Input: part model. Units: mm. Frame: model coordinates. Round coordinates to 2 decimals unless told otherwise and drop trailing zeros. Write each loop counter-clockwise with the first axis right and the second up, starting at its lowest first coordinate (ties: lowest second). Pieces come first, ordered by that corner, then holes. Notation, with made-up numbers: (36.5, 59) - (54.5, 59) arc R25 ccw to (54.5, 95) - close; hole circle Ø2 at (-18.75, 5). An arc over 180 degrees is marked (long way). Use one line per item in the form item = value.
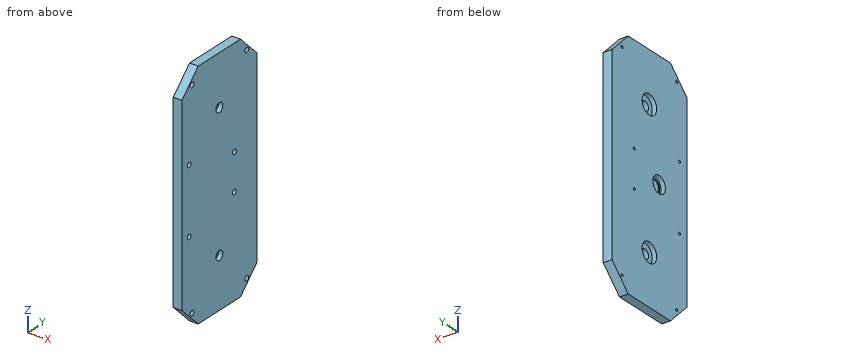
Autodesk Inventor part; units mm, degrees
ref_plane "YZ Plane" through (0, 0, 0) normal (1, 0, 0) x (0, 1, 0)
ref_plane "XZ Plane" through (0, 0, 0) normal (0, 1, 0) x (-1, 0, 0)
ref_plane "XY Plane" through (0, 0, 0) normal (0, 0, 1) x (1, 0, 0)
sketch "Sketch1" plane through (0, 0, 0) normal (1, 0, 0) x (0, 1, 0)
  line L0 (-57.5, 135) -> (57.5, 135)
  line L1 (57.5, 135) -> (57.5, -135)
  line L2 (57.5, -135) -> (-57.5, -135)
  line L3 (-57.5, -135) -> (-57.5, 135)
  line L4 (-57.5, 135) -> (57.5, -135) construction
  line L5 (57.5, 135) -> (-57.5, -135) construction
  circle A0 centre (0, 77.5) radius 5.3
  circle A1 centre (0, -77.5) radius 5.3
  circle A2 centre (0, 0) radius 5.3
  line L6 (0, 77.5) -> (0, -77.5) construction
  line L7 (51.5, -129) -> (51.5, 129)
  line L8 (51.5, 129) -> (-51.5, 129)
  line L9 (-51.5, 129) -> (-51.5, -129)
  line L10 (-51.5, -129) -> (51.5, -129)
  dimension "d0" = 155
  dimension "d1" = 10.6
  dimension "d2" = 270
  dimension "d3" = 115
  dimension "d4" = 6
extrude "Extrusion1" add sketch "Sketch1" along normal blind 10 contours L0 L1 L2 L3 | A2 | L10 L9 L8 L7
chamfer "Chamfer2" distance 25 angle 45 4 edges at (5, 57.5, -135) (5, -57.5, -135) (5, -57.5, 135) (5, 57.5, 135)
sketch "Sketch11" plane through (0, 0, 0) normal (-1, 0, 0) x (0, 0, 1)
  circle A0 centre (-77.5, 0) radius 5.3
  circle A1 centre (77.5, 0) radius 5.3
  circle A2 centre (-77.5, 0) radius 11.15
  circle A3 centre (77.5, 0) radius 11.15
  point P0 (0, 0)
  dimension "d41" = 22.3
extrude "Extrusion10" cut sketch "Sketch11" against normal blind 5 contours A0 | A1 | A2 | A3
sketch "Sketch12" plane through (0, 0, 0) normal (-1, 0, 0) x (0, 0, 1)
  circle A0 centre (0, -15) radius 9.65
  point P0 (0, 0)
  dimension "d44" = 15
  dimension "d45" = 19.3
extrude "Extrusion11" cut sketch "Sketch12" against normal blind 5
sketch "Sketch13" plane through (5, -15, 0) normal (-1, 0, 0) x (0, 0, 1)
  circle A0 centre (0, 0) radius 9.65
  circle A1 centre (0, 0) radius 7.5
  point P0 (0, 15)
  dimension "d48" = 15
extrude "Extrusion12" cut sketch "Sketch13" against normal blind 1 contours A1
sketch "Sketch14" plane through (10, 0, 0) normal (1, 0, 0) x (0, 0, -1)
  circle A0 centre (-119.5, 42) radius 1.5
  circle A1 centre (-119.5, -42) radius 1.5
  circle A2 centre (-37.6476, -46.4615) radius 1.5
  circle A3 centre (37.6476, -46.4615) radius 1.5
  circle A4 centre (-21.0923, 23.1558) radius 1.5
  circle A5 centre (21.0923, 23.1558) radius 1.5
  circle A6 centre (119.5, -42) radius 1.5
  circle A7 centre (119.5, 42) radius 1.5
  point P0 (0, 0)
extrude "Extrusion13" cut sketch "Sketch14" against normal through all
sketch "Sketch15" plane through (10, 0, 0) normal (1, 0, 0) x (0, 0, -1)
  circle A0 centre (-21.0923, 23.1558) radius 1.5
  circle A1 centre (119.5, -42) radius 1.5
  circle A2 centre (-119.5, -42) radius 1.5
  circle A3 centre (37.6476, -46.4615) radius 1.5
  circle A4 centre (-37.6476, -46.4615) radius 1.5
  circle A5 centre (-119.5, 42) radius 1.5
  circle A6 centre (21.0923, 23.1558) radius 1.5
  circle A7 centre (119.5, 42) radius 1.5
  line L0 (-135, 32.5) -> (-110, 57.5)
  line L1 (-135, 32.5) -> (-135, -32.5)
  line L2 (-110, -57.5) -> (-135, -32.5)
  line L3 (-110, -57.5) -> (110, -57.5)
  line L4 (135, -32.5) -> (110, -57.5)
  line L5 (135, -32.5) -> (135, 32.5)
  line L6 (110, 57.5) -> (135, 32.5)
  line L7 (110, 57.5) -> (-110, 57.5)
  circle A8 centre (-77.5, 0) radius 5.3
  circle A9 centre (77.5, 0) radius 5.3
  circle A10 centre (-119.5, 42) radius 2.9
  circle A11 centre (-119.5, -42) radius 2.9
  circle A12 centre (-37.6476, -46.4615) radius 2.9
  circle A13 centre (37.6476, -46.4615) radius 2.9
  circle A14 centre (119.5, -42) radius 2.9
  circle A15 centre (119.5, 42) radius 2.9
  circle A16 centre (21.0923, 23.1558) radius 2.9
  circle A17 centre (-21.0923, 23.1558) radius 2.9
  point P0 (0, 0)
  dimension "d53" = 5.8
extrude "Extrusion14" cut sketch "Sketch15" against normal blind 4 contours A0 | A1 | A2 | A3 | A4 | A5 | A6 | A7 | A10 | A11 | A12 | A13 | A14 | A15 | A16 | A17
properties part number "CAJA" material "Steel, Mild, Welded"
(1) Material intervals for L1, parallel to Z at x = 2.25, y = 10; L2, parallel to Y at x = 2.1, z = -77.5; L3, parallel to Y at x = 7.7, z = 77.5, sorted ascending.
Derived:
L1 = -135 to -82.43, -72.57 to 72.57, 82.43 to 135
L2 = -57.5 to -11.15, 11.15 to 57.5
L3 = -57.5 to -5.3, 5.3 to 57.5
(2) Cut plane C-C on x = 1.5. Count the separate pieces of the cut face and the enclosed holes in it, then the cut area to 3 significant figures.
Derived:
separate_pieces = 1
enclosed_holes = 11
area = 28,700 mm^2
(3) Cut plane B-B on z = 0. Output: boundary loops of the cut face in (x, y).
Derived:
outline = (0, -57.5) - (10, -57.5) - (10, 57.5) - (0, 57.5) - (0, -5.35) - (5, -5.35) - (5, -7.5) - (6, -7.5) - (6, -22.5) - (5, -22.5) - (5, -24.65) - (0, -24.65) - close
(4) Cut plane A-A on y = 0. Output: boundary loops of the cut face in (x, z).
Derived:
outline = (0, -135) - (10, -135) - (10, -82.8) - (5, -82.8) - (5, -88.65) - (0, -88.65) - close; (0, -66.35) - (5, -66.35) - (5, -72.2) - (10, -72.2) - (10, 72.2) - (5, 72.2) - (5, 66.35) - (0, 66.35) - close; (0, 88.65) - (5, 88.65) - (5, 82.8) - (10, 82.8) - (10, 135) - (0, 135) - close
(5) First-contact query: pin 1 Ø3 at (y, z) = (-42, -118.5) entering from +X; pin 2 Ø12 at (y, z) = (-16, -1) entering from -X; pin 3 Ø6.5 at (y, z) = (-0.5, 75) entering from -X. Flat tips, straight axial feed; report the tip coordinate or a pass-through.
Derived:
pin_1 = 6
pin_2 = 6
pin_3 = 5
